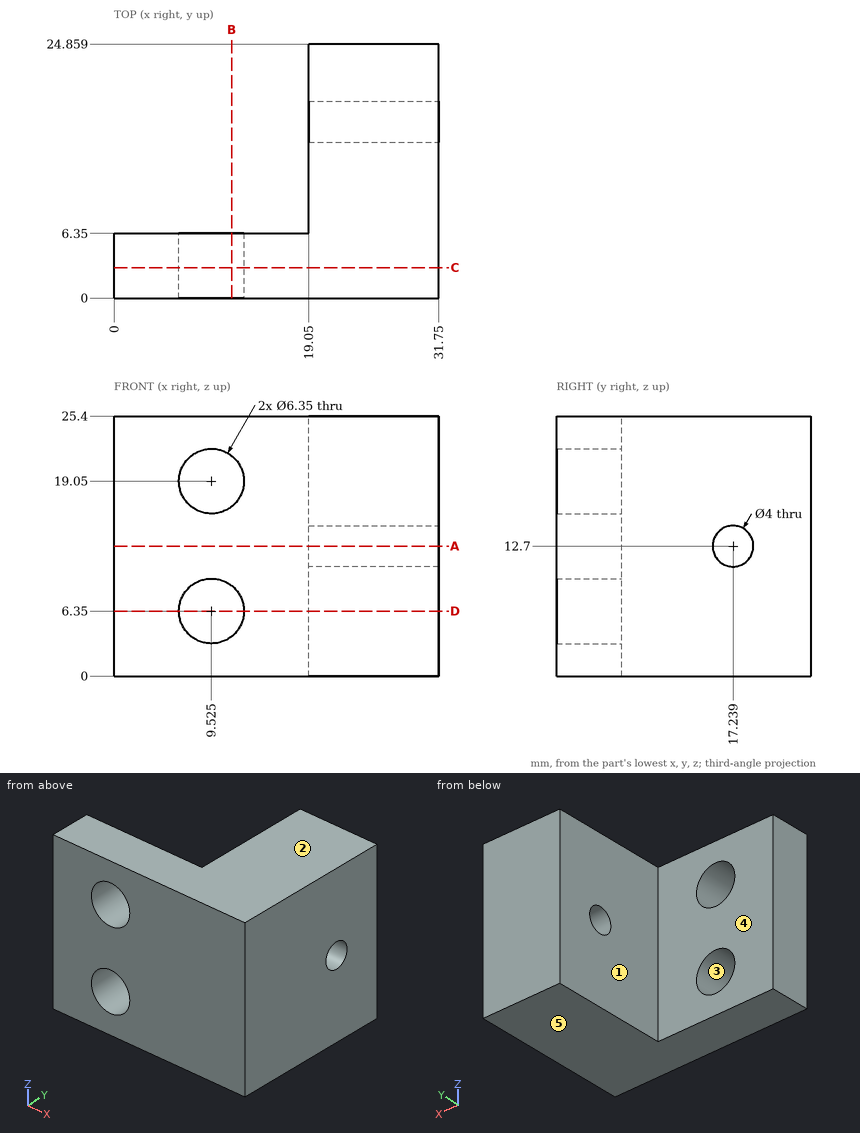
Job drawing, mm, ordinate dimensions from the low corner. One solid piece. A direction names the side the tool comes from. Coordinates: 2 decimals unless noted, no trailing zeros. Write each loop counter-clockwise with the first axis right and the second up, starting at its lowest first coordinate (ties: lowest second). Pieces come first, ordered by that corner, then holes. Notation, with made-up numbers: M 50,72 L 61,72 A31 cw 61,96 Z; hole C 22,25.25 d7. An arc over 180 degrees is marked long. Answer as a JSON object with one key per item and string values. Group by question number.
1) Tool access for the marked faces 4 and 5: list every direction of +Z, -Z, +X, -X, +Y, -Y with a clear straight run to the whole face (end or side of a thin tool).
2) Pin check, flat tips, straight feed: pin 1 Ø8.5 at (x, z) = (9.525, 6.35) entering from +Y; pin 2 Ø6.5 at (y, z) = (17.239, 12.7) entering from +X; pin 3 Ø5 at (y, z) = (18.5, 15.5) entering from -X. Stop position of each tip, or through.
3) Wall check: line 1 (Z direction, x = 7.5, y = 2.25); line 2 (X direction, y = 2.25, z = 6.35); line 3 (Y direction, x = 29, z = 12.7). Give the ranges that are in metal, low to high. Write a range as from..to.
4) Saw through at D-D (z = 6.35). Write the cut outline in (x, y), plus the area to 3 significant figures.
5) Saw through at C-C (y = 3). Write the cut outline in (x, z) (3 decimals), plus the area to 3 significant figures.
6) Saw through at A-A (z = 12.7). Write the cut outline in (x, y), plus the area to 3 significant figures.
7) Saw through at B-B (x = 11.5). Write the cut outline in (y, z), plus the area to 3 significant figures.
8) Mould opens along X. For the marked faces 1, 2 and 3 say: +X half, -X half, draft (parallel to the pull), parting line (faces both ways), or undercut.
Values follow:
{
 "1": {"face 4": "+Z, -Z, -X, +Y", "face 5": "-Z, +X, -X, +Y, -Y"},
 "2": {"pin 1": "stops at y = 6.35", "pin 2": "stops at x = 31.75", "pin 3": "stops at x = 19.05"},
 "3": {"line 1": "z = 0..3.9, 8.8..16.6, 21.5..25.4", "line 2": "x = 0..6.35, 12.7..31.75", "line 3": "y = 0..15.24, 19.24..24.86"},
 "4": {"outline": "M 0,0 L 6.35,0 L 6.35,6.35 L 0,6.35 Z; M 12.7,0 L 31.75,0 L 31.75,24.86 L 19.05,24.86 L 19.05,6.35 L 12.7,6.35 Z", "area": "396 mm2"},
 "5": {"outline": "M 0,0 L 31.75,0 L 31.75,25.4 L 0,25.4 Z; hole C 9.525,6.35 d6.35; hole C 9.525,19.05 d6.35", "area": "743 mm2"},
 "6": {"outline": "M 0,0 L 31.75,0 L 31.75,15.24 L 19.05,15.24 L 19.05,6.35 L 0,6.35 Z; M 19.05,19.24 L 31.75,19.24 L 31.75,24.86 L 19.05,24.86 Z", "area": "386 mm2"},
 "7": {"outline": "M 0,0 L 6.35,0 L 6.35,3.86 L 0,3.86 Z; M 0,8.84 L 6.35,8.84 L 6.35,16.56 L 0,16.56 Z; M 0,21.54 L 6.35,21.54 L 6.35,25.4 L 0,25.4 Z", "area": "98.1 mm2"},
 "8": {"face 1": "-X half", "face 2": "draft", "face 3": "undercut"}
}
